Could you check a few things on this drawing? It's one solid part, dimensions in mm from its lowest x, y, z. A direction names the side the tool comes from. Give positions to 0.01 mm unless a question says otherwise; leave off trailing zeros. Loops run counter-clockwise (first coordinate to the right, second up) from the corner with the lowest first, then second, coordinate; pieces in that order, holes last. Notation, with made-up numbers: (9, -21) - (66, -21) arc R11 cw to (66, -16) - close; hole circle Ø5 at (-8, -35). An arc over 180 degrees is marked (long way). Put each result on its own line as item: value. Start each with the question number.
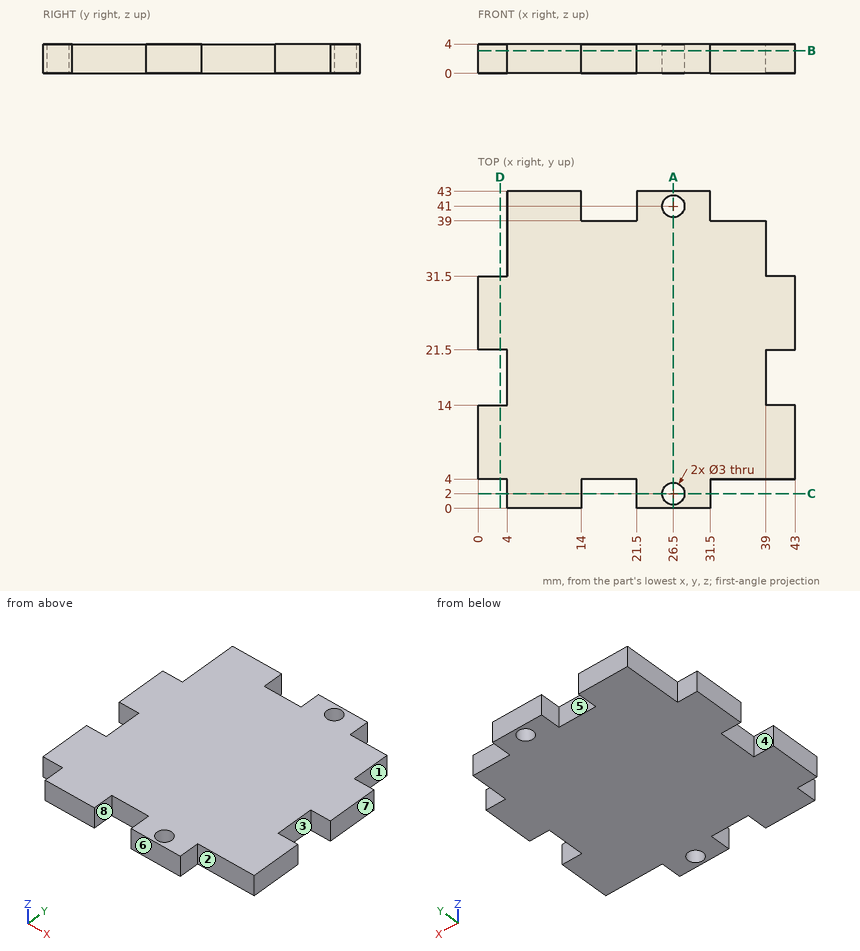
1) Suppose I cut it at D-D on x = 3. Please give me the cut outline in (y, z).
2) I need wall thicknesses on line 1 (Y direction, x = 26.5, z = 1.65); line 2 (Y direction, x = 37, z = 2.5); line 3 (Y direction, x = 3, z = 1.5). Which ranges of each line are inside material? Lowest first, please.
3) Suppose I cut it at C-C on y = 2. Please give me the cut outline in (x, z), plus the area to 3 significant figures.
4) Suppose I cut it at B-B on z = 3.1. Give the number of separate pieces and of enclosed holes in the cut face, plus the area to 3 significant figures.
5) I'm going to push flat-ended pins straight in: P1, Ø1.2, axis at x = 41, z = 2, coming from the +Y side; P2, Ø1.2, axis at y = 39.5, z = 2.5, coming from the -X side; P3, Ø2, axis at x = 40.5, z = 1, coming from the -Y side; P4, Ø2.5, axis at x = 26.5, y = 2, coming from the +Z side. Where does each tip first touch, or does it pass through?
6) Thinking about a two-plate mould opening in X: for the marked faces 5, 6, 7 and 8, which applies, pulls with the +X half, pulls with the -X half, needs draft (parallel to the pull), parting line crosses it, or undercut?
7) Which directions (+Z, -Z, +X, -X, +Y, -Y) give clear straight access to the entire face, cutting with the end or side of a thin tool? Please do the marked faces 1, 2, 3 and 4.
8) Suppose I cut it at A-A on x = 26.5. Please give me the cut outline in (y, z).
Ans:
1. outline: (4, 0) - (14, 0) - (14, 4) - (4, 4) - close; (21.5, 0) - (31.5, 0) - (31.5, 4) - (21.5, 4) - close
2. line 1: y = 0 to 0.5, 3.5 to 39.5, 42.5 to 43
2. line 2: y = 4 to 39
2. line 3: y = 4 to 14, 21.5 to 31.5
3. outline: (4, 0) - (14, 0) - (14, 4) - (4, 4) - close; (21.5, 0) - (25, 0) - (25, 4) - (21.5, 4) - close; (28, 0) - (31.5, 0) - (31.5, 4) - (28, 4) - close
3. area: 68.0 mm²
4. separate pieces: 1
4. enclosed holes: 2
4. area: 1,530 mm²
5. P1: stops at y = 31.5
5. P2: stops at x = 4
5. P3: stops at y = 4
5. P4: passes through
6. face 5: undercut
6. face 6: needs draft
6. face 7: pulls with the +X half
6. face 8: undercut
7. face 1: +Z, -Z, +X, +Y
7. face 2: +Z, -Z, +X, -Y
7. face 3: +Z, -Z, +X
7. face 4: +Z, -Z, -X
8. outline: (0, 0) - (0.5, 0) - (0.5, 4) - (0, 4) - close; (3.5, 0) - (39.5, 0) - (39.5, 4) - (3.5, 4) - close; (42.5, 0) - (43, 0) - (43, 4) - (42.5, 4) - close
